Could you check a few things on this model? Use its own coordinates, in mm. A direction names the side the tool comes from. Give positions to 0.01 mm unless a question says otherwise; leave off trailing zeros. Loops run counter-clockwise (first coordinate to the right, second up) from the corner with the lowest first, then second, coordinate; pieces in that order, holes last. Notation, with made-up numbers: (-9, 66) - (39, 66) arc R17 cw to (39, 82) - close; hole circle Ø10 at (12.5, 22). An arc over 180 degrees is marked (long way). One line per item, written item: value. Start each with the question number.
Q1. If we mould it in two halves opening along Y, with no side actions, what happens to faces 4 (the face through (-0.02, 3.86, -0.01)), 5 (the face through (-3.495, -1.64, -0.006)), 6 (the face through (-0.276, 8.377, -0.006)), 7 (the face through (-2.143, 4.327, -0.006))? For each: released by +Y, released by -Y, zero draft, split by the parting line, or undercut.
Q2. I want a section at D-D (y = 4.5). Please give me the cut outline in (x, z).
Q3. If I drill on line 1 (X direction, y = 4.25, z = 0.25); line 2 (X direction, y = 4.5, z = -0.2); line 3 (Y direction, x = 5.75, z = -0.2), over which ranges is the centre line in solid material (lowest first)? Write a range as from..to.
Q4. For faces 1 (the face through (2.143, 4.327, -0.006)), 2 (the face through (-3.134, -4.459, -0.006)), 3 (the face through (-0.1, 4.4, 0.444)), which set-ups out of +Z, -Z, +X, -X, +Y, -Y let a thin tool reach every point of the face, with its end or its side?
Q5. I want a section at A-A (y = -3.75). Please give me the cut outline in (x, z), then the cut area to 3 significant figures.
Q6. I want a section at C-C (x = 4.25). Please give me the cut outline in (y, z).
Q7. I'm going to push a flat-ended pin straight in: P1, Ø1, axis at x = 1.5, y = 1, coming from the -Z side. Where does the tip first touch, or does it pass through?
Q8. I want a section at B-B (z = -0.1). Please give me the cut outline in (x, y).
Autodesk Inventor part; units mm, degrees
ref_plane "YZ Plane" through (0, 0, 0) normal (1, 0, 0) x (0, 1, 0)
ref_plane "XZ Plane" through (0, 0, 0) normal (0, 1, 0) x (-1, 0, 0)
ref_plane "XY Plane" through (0, 0, 0) normal (0, 0, 1) x (1, 0, 0)
sketch "Sketch1" plane through (0, 0, 0) normal (0, 0, 1) x (1, 0, 0)
  line L0 (-11.7348, 0) -> (11.7348, 0)
  line L1 (0, -9.2893) -> (0, 11.3272)
  arc A0 (5.9648, -5.8889) -> (-5.9648, -5.8889) centre (0, 0) ccw
  arc A1 (-5.9648, -5.8889) -> (-4.0207, -5.7251) centre (-5.061, -4.9966) ccw
  arc A2 (4.0207, -5.7251) -> (5.9648, -5.8889) centre (5.061, -4.9966) ccw
  line L2 (0, 0) -> (-6.8661, 4.8077) construction
  line L3 (0, 0) -> (6.8661, 4.8077) construction
  line L4 (4.0207, -5.7251) -> (2.2225, -3.1569)
  line L5 (-4.0207, -5.7251) -> (-2.2225, -3.1569)
  line L6 (1.6581, 3.4866) -> (2.642, 5.1906)
  line L7 (-1.6581, 3.4866) -> (-2.642, 5.1906)
  line L8 (-3.8434, 0.3656) -> (-5.7812, 0.7073)
  line L9 (3.8434, 0.3656) -> (5.7812, 0.7073)
  arc A3 (-3.274, 5.3751) -> (-6.1707, 1.2381) centre (-0.7559, 0.5293) ccw
  arc A4 (6.1707, 1.2381) -> (3.274, 5.3751) centre (0.7559, 0.5293) ccw
  arc A5 (-2.642, 5.1906) -> (-3.274, 5.3751) centre (-3.0544, 4.9525) ccw
  arc A6 (-6.1707, 1.2381) -> (-5.7812, 0.7073) centre (-5.6985, 1.1763) ccw
  arc A7 (3.274, 5.3751) -> (2.642, 5.1906) centre (3.0544, 4.9525) ccw
  arc A8 (5.7812, 0.7073) -> (6.1707, 1.2381) centre (5.6985, 1.1763) ccw
  arc A9 (-3.8434, 0.3656) -> (-2.2225, -3.1569) centre (0, 0) ccw
  arc A10 (2.2225, -3.1569) -> (3.8434, 0.3656) centre (0, 0) ccw
  arc A11 (1.6581, 3.4866) -> (-1.6581, 3.4866) centre (0, 0) ccw
  point P0 (2.8602, 5.5686)
  point P1 (-2.8602, 5.5686)
  point P2 (-6.211, 0.7831)
  point P3 (6.211, 0.7831)
  dimension "d19" = 1.27
  dimension "d30" = 8.382
  dimension "d35" = 35
  dimension "d36" = 35
  dimension "d37" = 4.445
  dimension "d38" = 30
  dimension "d39" = 2.4041
  dimension "d40" = 0.4763
  dimension "d41" = 3.8608
  dimension "d42" = 3.8608
  dimension "d43" = 3.8608
  dimension "d45" = 3.81
  dimension "d46" = 5.461
extrude "Extrusion2" add sketch "Sketch1" along normal mid plane 0.889 contours A0 L1 A11 L7 A5 A3 A6 L8 A9 L0 | L0 A9 L5 A1 A0 | A0 L0 A10 L9 A8 A4 A7 L6 A11 L1 | A0 A2 L4 A10 L0
properties part number "e-clip" material "Steel, Mild"
Worked answers:
1. face 4: released by -Y
1. face 5: undercut
1. face 6: split by the parting line
1. face 7: undercut
2. outline: (-7.07, -0.44) - (-4.51, -0.44) - (-4.51, 0.44) - (-7.07, 0.44) - close; (-2.24, -0.44) - (2.24, -0.44) - (2.24, 0.44) - (-2.24, 0.44) - close; (4.51, -0.44) - (7.07, -0.44) - (7.07, 0.44) - (4.51, 0.44) - close
3. line 1: x = -7.22..-4.75, -2.1..2.1, 4.75..7.22
3. line 2: x = -7.07..-4.51, -2.24..2.24, 4.51..7.07
3. line 3: y = -6.06..0.7, 2.74..6.1
4. face 1: +Z, -Z
4. face 2: +Z, -Z, -Y
4. face 3: +Z, +X, -X, +Y, -Y
5. outline: (-7.5, -0.44) - (-2.64, -0.44) - (-2.64, 0.44) - (-7.5, 0.44) - close; (2.64, -0.44) - (7.5, -0.44) - (7.5, 0.44) - (2.64, 0.44) - close
5. area: 8.64 mm²
6. outline: (-5.97, -0.44) - (0.44, -0.44) - (0.44, 0.44) - (-5.97, 0.44) - close; (4.73, -0.44) - (7.22, -0.44) - (7.22, 0.44) - (4.73, 0.44) - close
7. P1: passes through
8. outline: (-6.17, 1.24) arc R5.46 cw to (-3.27, 5.38) arc R0.48 cw to (-2.64, 5.19) - (-1.66, 3.49) arc R3.86 cw to (1.66, 3.49) - (2.64, 5.19) arc R0.48 cw to (3.27, 5.38) arc R5.46 cw to (6.17, 1.24) arc R0.48 cw to (5.78, 0.71) - (3.84, 0.37) arc R3.86 cw to (2.22, -3.16) - (4.02, -5.73) arc R1.27 ccw to (5.96, -5.89) arc R8.38 ccw (long way) to (-5.96, -5.89) arc R1.27 ccw to (-4.02, -5.73) - (-2.22, -3.16) arc R3.86 cw to (-3.84, 0.37) - (-5.78, 0.71) arc R0.48 cw to start
